```python
from build123d import *

# Parameters (mm, degrees)
SKETCH1_W      = 6
SKETCH1_H      = 12.3
EXTRUDE1_DEPTH = 309.396319693
HOLE1_D        = 6
CHAMFER1_SIZE  = 1
SKETCH5_R      = 1.1
EXTRUDE3_DEPTH = 80
SKETCH6_R      = 4.2
EXTRUDE4_DEPTH = 10
EXTRUDE4_DRAFT = -15


with BuildPart() as part:
    # Sketch1 → Revolve1 (revolve)
    with BuildSketch(Plane(origin=(0, 295, 0), x_dir=(-1, 0, 0), z_dir=(0, 1, 0))):
        with Locations((-63, 12.85)):
            Rectangle(SKETCH1_W, SKETCH1_H)
    revolve(axis=Axis((60, 295, 6.7), (0, 0, 1)))

    # Sketch2 → Extrude1 (cut, through all)
    with BuildSketch(Plane(origin=(0, 0, 6.7), x_dir=(-1, 0, 0), z_dir=(0, 0, -1))):
        with BuildLine():
            Line((-61, 300.916079783), (-61, 299.9))
            Line((-61, 299.9), (-59, 299.9))
            Line((-59, 299.9), (-59, 300.916079783))
            ThreePointArc((-59, 300.916079783), (-60, 301), (-61, 300.916079783))
        make_face()
    extrude(amount=-EXTRUDE1_DEPTH, mode=Mode.SUBTRACT)

    # Hole1 (through all)
    with Locations(Plane(origin=(0, 0, 6.7), x_dir=(-1, 0, 0), z_dir=(0, 0, -1))):
        with Locations((-60, 295)):
            Hole(HOLE1_D / 2)

    # Chamfer1
    chamfer1_edges = [part.edges().sort_by_distance(p)[0] for p in [
        (60, 289, 19),
    ]]
    chamfer(chamfer1_edges, length=CHAMFER1_SIZE)

    # Sketch5 → Extrude3 (cut)
    with BuildSketch(Plane(origin=(0, 0, 0), x_dir=(0, 0, -1), z_dir=(1, 0, 0))):
        with Locations(Location((-14, 294.95, 0), (0, 0, 180))):
            Circle(SKETCH5_R)
    extrude(amount=EXTRUDE3_DEPTH, mode=Mode.SUBTRACT)


with BuildPart() as extrude4_tool:
    # Sketch6 → Extrude4 (with draft: the straight prism first)
    with BuildSketch(Plane.XY.offset(19)):
        with Locations((60, 295)):
            Circle(SKETCH6_R)
    extrude(amount=-EXTRUDE4_DEPTH)
    # Extrude4: the draft: its side faces are tilted about the plane it starts from
    extrude4_sides = [extrude4_tool.faces().sort_by_distance(p)[0] for p in [
        (55.8, 295, 14),
    ]]
    draft(extrude4_sides, Plane.XY.offset(19), EXTRUDE4_DRAFT)


with BuildPart() as part_1:
    add(part.part)

    # Extrude4: cut by extrude4_tool
    add(extrude4_tool.part, mode=Mode.SUBTRACT)


solid = part_1.part
```
CAD build for the part. Positions are in the model's coordinates, mm. A direction names the side the tool comes from. Coordinates: 2 decimals unless noted, no trailing zeros. Loops run counter-clockwise (first coordinate to the right, second up) from the corner with the lowest first, then second, coordinate; pieces in that order, holes last. Notation, with made-up numbers: (77, 89.25) - (95, 89.25) arc R16 ccw to (95, 112.25) - close; hole circle Ø1 at (63, -1). An arc over 180 degrees is marked (long way). Use CSV: the item, a comma, the result in double quotes. Start each with the question number.
Q1. Cut at C-C, the plane z = 8.5. List the corners of the cut face in (x, y).
Q2. Cut at B-B, the plane z = 14.75. List the corners of the cut face in (x, y), then the cut area to 3 significant figures.
Q3. Cut at D-D, the plane y = 295.25. State how many separate pieces and enclosed holes the cut face has, then the cut area to 3 significant figures.
Q4. 3-axis set-ups, long thin cutter, end or side, ignore diameter. For faces 1 (the conical face through (63.09, 293.72, 15.8)), 2 (the flat face through (61, 300.4, 12.8)): which of +Z, -Z, +X, -X, +Y, -Y reach the whole face in a straight line?
Q5. Probe probe 1 along Z at (x, y) = (64.3, 294.95); probe 2 along Y at (x, z) = (62.75, 9.25); probe 3 along Y at (x, z) = (63.5, 13). List the from-to ranges inside material, lowest first. Write a range as from..to.
Q6. Two-plate mould, pull along X, no slides. Class faces 3 (the cylindrical face through (55.6, 294.9, 12.9)), 4 (the cylindrical face through (62.77, 293.85, 10.67)), 5 (the cylindrical face through (60, 289, 12)): +X half, -X half, draft (parallel to the pull), parting line (faces both ways), or undercut.
Q7. Cut at A-A, the plane x = 60. List the corners of the cut face in (y, z).
Q8. Drop flat-ended pins along their axis: P1, Ø4, axis at x = 56, z = 14.5, coming from the -Y side; P2, Ø1.1, axis at y = 300.5, z = 10, coming from the +X side; P3, Ø6, axis at x = 55.5, z = 17.5, coming from the -Y side. Give the stop position or say it passes through.
Here are the results:
1,outline,"(59, 299.9) - (59, 300.92) arc R6 ccw (long way) to (61, 300.92) - (61, 299.9) - close; hole circle Ø6 at (60, 295)"
2,outline,"(54.05, 295.75) - (57.03, 295.75) arc R3.06 cw to (62.97, 295.75) - (65.95, 295.75) arc R6 ccw to (61, 300.92) - (61, 299.9) - (59, 299.9) - (59, 300.92) arc R6 ccw to start; (54.06, 294.15) arc R6 ccw to (65.94, 294.15) - (62.94, 294.15) arc R3.06 cw to (57.06, 294.15) - close"
2,area,"72.0 mm2"
3,separate pieces,"4"
3,enclosed holes,"0"
3,area,"54.9 mm2"
4,face 1,"+Z"
4,face 2,"+Z, -Z, +Y"
5,probe 1,"6.7..12.9, 15.1..19"
5,probe 2,"289.67..293.8, 296.2..300.33"
5,probe 3,"290.13..294.49, 295.41..299.87"
6,face 3,"draft"
6,face 4,"undercut"
6,face 5,"parting line"
7,outline,"(289, 6.7) - (292, 6.7) - (292, 14.52) - (290.8, 19) - (290, 19) - (289, 18) - close; (298, 6.7) - (299.9, 6.7) - (299.9, 19) - (299.2, 19) - (298, 14.52) - close"
8,P1,"y = 289.34"
8,P2,"x = 63.39"
8,P3,"y = 289.19"
